from build123d import *

# Parameters (mm, degrees)
SKETCH1_R           = 11.1633
SKETCH1_R_2         = 9.1313
BOSS_EXTRUDE1_DEPTH = 81.28
BOSS_EXTRUDE2_DEPTH = 0.889
CIRPATTERN1_COUNT   = 3
SKETCH3_R           = 9.1313
SKETCH3_R_2         = 6.35
BOSS_EXTRUDE3_DEPTH = 3.175
BOSS_EXTRUDE4_START = -0.461027
SKETCH5_W           = 9.525
SKETCH5_H           = 6.35
BOSS_EXTRUDE4_DEPTH = 4.271027
BOSS_EXTRUDE5_DEPTH = 9.525
SKETCH7_R           = 1.905
CUT_EXTRUDE1_DEPTH  = 9.525


with BuildPart() as part:
    # Sketch1 → Boss-Extrude1 (new body)
    with BuildSketch(Plane(origin=(0, 0, 0), x_dir=(1, 0, 0), z_dir=(0, 1, 0))):
        with Locations(Location((0, 0, 0), (0, 0, 270))):
            Circle(SKETCH1_R)
        with Locations(Location((0, 0, 0), (0, 0, 270))):
            Circle(SKETCH1_R_2, mode=Mode.SUBTRACT)
    extrude(amount=BOSS_EXTRUDE1_DEPTH)

    # Sketch2 → Boss-Extrude2 (add, symmetric)
    with BuildSketch(Plane.XY):
        Polygon((11.1633, 0), (9.1313, 0), (9.1313, 20.32), (11.1633, 20.32), (41.6433, -3.408032613), (41.6433, -8.103225478), (32.1183, -8.103225478), align=None)
    boss_extrude2 = extrude(amount=BOSS_EXTRUDE2_DEPTH, both=True)

    # CirPattern1: Boss-Extrude2 ×3 about axis
    cirpattern1_axis = Axis((0, 0, 0), (0, 1, 0))
    for i in range(1, CIRPATTERN1_COUNT):
        add(boss_extrude2.rotate(cirpattern1_axis, i * 360 / CIRPATTERN1_COUNT))

    # Sketch3 → Boss-Extrude3 (add)
    with BuildSketch(Plane(origin=(0, 63.5, 0), x_dir=(1, 0, 0), z_dir=(0, 1, 0))):
        with Locations(Location((0, 0, 0), (0, 0, 270))):
            Circle(SKETCH3_R)
        with Locations(Location((0, 0, 0), (0, 0, 270))):
            Circle(SKETCH3_R_2, mode=Mode.SUBTRACT)
    extrude(amount=BOSS_EXTRUDE3_DEPTH)

    # Sketch5 → Boss-Extrude4 (add)
    with BuildSketch(Plane(origin=(5.58165, 0, -9.66770139), x_dir=(0, -1, 0), z_dir=(0.500000000000001, 0, -0.866025403784438)).offset(BOSS_EXTRUDE4_START)):
        with Locations((-51.1175, 0)):
            Rectangle(SKETCH5_W, SKETCH5_H)
    extrude(amount=BOSS_EXTRUDE4_DEPTH)

    # Sketch6 → Boss-Extrude5 (add)
    with BuildSketch(Plane(origin=(0, 55.88, 0), x_dir=(1, 0, 0), z_dir=(0, 1, 0))):
        with BuildLine():
            Line((4.737019343, 14.554758178), (10.236280657, 11.379758178))
            ThreePointArc((10.236280657, 11.379758178), (9.07415, 15.716888836), (4.737019343, 14.554758178))
        make_face()
    extrude(amount=-BOSS_EXTRUDE5_DEPTH)

    # Sketch7 → Cut-Extrude1 (cut)
    with BuildSketch(Plane(origin=(0, 55.88, 0), x_dir=(1, 0, 0), z_dir=(0, 1, 0))):
        with Locations(Location((7.48665, 12.967258178, 0), (0, 0, 270))):
            Circle(SKETCH7_R)
    extrude(amount=-CUT_EXTRUDE1_DEPTH, mode=Mode.SUBTRACT)


solid = part.part
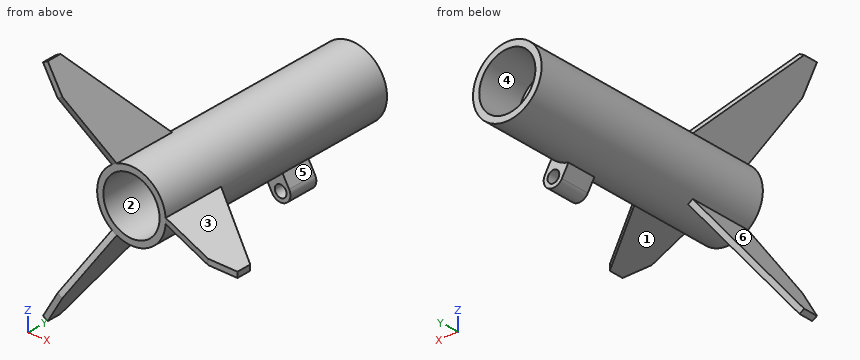
Input: part model. Units: mm. Frame: model coordinates. Face numbers are marked on the shaded views. A direction names the side the tool comes from. Give positions to 0.01 mm unless a question says otherwise; leave off trailing zeros. Order: outer loops, then holes, each group sorted by start corner. A loop starts at its lowest first (then second) coordinate and runs counter-clockwise, first axis right, second up. Notation, with made-up numbers: (23.5, 10) - (80.5, 10) arc R19 ccw to (80.5, 47) - close; hole circle Ø1 at (81.5, 7.5). An arc over 180 degrees is marked (long way). Answer as a JSON object with one key per item and string values. Group by question number.
Q1. First-contact query: pin 1 Ø5 at (x, y) = (-1, 5.5) entering from +Z; pin 2 Ø4 at (y, z) = (54, 6) entering from -X; pin 3 Ø2 at (x, y) = (3.5, 66) entering from +Z. Flat tips, straight axial feed; report the tip coordinate or a pass-through.
Q2. Mould query, pull axis Z, two halves, no side actions, for the marked faces 1, 2 and 3. Classes: pulls with the +Z half, pulls with the -Z half, needs draft (parallel to the pull), parting line crosses it, or undercut.
Q3. Set-up query: the marked faces 4, 5 and 6. Return all of +Z, -Z, +X, -X, +Y, -Y with unobstructed straight access to the full face (end or side cutting, diameter ignored); none if empty.
Q4. Cut plane D-D, the plane x = 15.5. Output: boundary loops of the cut face in (y, z).
Q5. Line query: probe 1 along Z at (x, y) = (0, 16); probe 2 along X at (y, z) = (36.5, -5.5); probe 3 along X at (y, z) = (19, 0). Output: solid intervals per line, ascending.
Q6. Cut plane B-B, the plane y = 18. Output: boundary loops of the cut face in (x, z).
Q7. Cut plane A-A, the plane x = 0. Output: boundary loops of the cut face in (y, z) (3 decimals), then the cut area to 3 significant figures.
Q8. Cut plane C-C, the plane z = 15.5. Output: boundary loops of the cut face in (x, y).
Results:
{
 "1": {"pin 1": "z = 11.16", "pin 2": "x = -10.42", "pin 3": "z = 10.88"},
 "2": {"face 1": "pulls with the -Z half", "face 2": "undercut", "face 3": "pulls with the +Z half"},
 "3": {"face 4": "+Y", "face 5": "+X, +Y, -Y", "face 6": "-X, +Y, -Y"},
 "4": {"outline": "(-1.68, -0.89) - (16.94, -0.89) - (16.94, 0.89) - (-1.68, 0.89) - close"},
 "5": {"probe 1": "-11.16 to -9.13, 9.13 to 11.16", "probe 2": "-9.71 to -7.29, 7.29 to 9.71", "probe 3": "-11.16 to -9.13, 9.13 to 12.86"},
 "6": {"outline": "(-7.84, -11.8) - (-6.3, -12.69) - (-4.79, -10.08) arc R11.16 ccw to (11.13, -0.89) - (14.14, -0.89) - (14.14, 0.89) - (11.13, 0.89) arc R11.16 ccw to (-4.79, 10.08) - (-6.3, 12.69) - (-7.84, 11.8) - (-6.33, 9.19) arc R11.16 ccw to (-6.33, -9.19) - close; hole circle Ø18.26 at (0, 0)"},
 "7": {"outline": "(0, -11.163) - (81.28, -11.163) - (81.28, -9.131) - (66.675, -9.131) - (66.675, -6.35) - (63.5, -6.35) - (63.5, -9.131) - (0, -9.131) - close; (0, 9.131) - (63.5, 9.131) - (63.5, 6.35) - (66.675, 6.35) - (66.675, 9.131) - (81.28, 9.131) - (81.28, 11.163) - (0, 11.163) - close", "area": "348 mm^2"},
 "8": {"outline": "(-9.98, -2.8) - (-7.92, -2.41) - (-7.92, 15.48) - (-9.98, 14.68) - close"}
}
